Verification items for the finished model (mm, model axes). Coordinates: 2 decimals unless noted, no trailing zeros. Order: outer loops, then holes, each group sorted by start corner. A loop starts at its lowest first (then second) coordinate and runs counter-clockwise, first axis right, second up. Notation, with made-up numbers: (-17.5, 88.25) -> (5.5, 88.25) arc R15 ccw to (5.5, 115.25) -> close; hole circle Ø5 at (29, 25). An arc over 180 degrees is marked (long way). Use CSV: the item, a comma, the result in double quotes. Start each with the question number.
1) Scan lines: line 1 along X through (y, z) = (-20, 2.5); line 2 along Y through (x, z) = (0, 1.75); line 3 along X through (y, z) = (-8, 7.5). Record each from-to range of solid material in increasing order.
2) Go/stop test with flat-tipped pins: pin 1 (4 mm diameter, centred on x = 2.5, y = -19, fed in from +Z); pin 2 (5 mm diameter, centred on y = -15.5, z = 4.5, fed in from +X); pin 3 (6.5 mm diameter, centred on x = 1.5, y = 0, fed in from +Z); pin 4 (2 mm diameter, centred on x = 0, y = 0, fed in from +Z). Record where each tip stops, or that it passes through.
3) Sectioned sample at B-B on z = 3.5. Record the boundary of the cut face in (x, y).
from build123d import *
from OCP.BRepFilletAPI import BRepFilletAPI_MakeChamfer

# Parameters (mm, degrees)
SKETCH1_R                      = 30
SKETCH1_R_2                    = 28
SKETCH1_R_3                    = 4
BOSS_EXTRUDE1_DEPTH            = 2
BOSS_EXTRUDE2_START            = 8
SKETCH1_3_R                    = 4
BOSS_EXTRUDE2_DEPTH            = 8
BOSS_EXTRUDE3_START            = 28
SKETCH1_4_R                    = 30
BOSS_EXTRUDE3_DEPTH            = 28
CHAMFER1_SIZE2                 = 20
CHAMFER1_SIZE                  = 24
CIRPATTERN1_COUNT              = 4
CHAMFER1_OF_CIRPATTERN1_SIZE   = 24
CHAMFER1_OF_CIRPATTERN1_SIZE_2 = 20


with BuildPart() as part:
    # Sketch1 → Boss-Extrude1 (new body)
    # profile 1 of 6: a face of its own
    with BuildSketch(Plane.XY):
        Circle(SKETCH1_R)
        Circle(SKETCH1_R_2, mode=Mode.SUBTRACT)
    # profile 2 of 6: a face of its own
    with BuildSketch(Plane.XY):
        with BuildLine():
            Line((-0.75, 27.989953555), (-0.75, 3.929058411))
            ThreePointArc((-0.75, 3.929058411), (0, 4), (0.75, 3.929058411))
            Line((0.75, 3.929058411), (0.75, 27.989953555))
            ThreePointArc((0.75, 27.989953555), (0, 28), (-0.75, 27.989953555))
        make_face()
    # profile 3 of 6: a face of its own
    with BuildSketch(Plane.XY):
        with BuildLine():
            ThreePointArc((4, 0), (-2.549509757, -3.082207001), (-0.75, 3.929058411))
            Line((-0.75, 3.929058411), (-0.75, 27.989953555))
            ThreePointArc((-0.75, 27.989953555), (-19.532024985, -20.062402648), (28, 0))
            ThreePointArc((28, 0), (20.062402648, 19.532024985), (0.75, 27.989953555))
            Line((0.75, 27.989953555), (0.75, 3.929058411))
            ThreePointArc((0.75, 3.929058411), (3.082207001, 2.549509757), (4, 0))
        make_face()
    # profile 4 of 6: a face of its own
    with BuildSketch(Plane.XY):
        with BuildLine():
            ThreePointArc((4, 0), (-2.549509757, -3.082207001), (-0.75, 3.929058411))
            Line((-0.75, 3.929058411), (-0.75, 27.989953555))
            ThreePointArc((-0.75, 27.989953555), (-19.532024985, -20.062402648), (28, 0))
            ThreePointArc((28, 0), (20.062402648, 19.532024985), (0.75, 27.989953555))
            Line((0.75, 27.989953555), (0.75, 3.929058411))
            ThreePointArc((0.75, 3.929058411), (3.082207001, 2.549509757), (4, 0))
        make_face()
    # profile 5 of 6: a face of its own
    with BuildSketch(Plane.XY):
        with BuildLine():
            Line((-0.75, 27.989953555), (-0.75, 3.929058411))
            ThreePointArc((-0.75, 3.929058411), (0, 4), (0.75, 3.929058411))
            Line((0.75, 3.929058411), (0.75, 27.989953555))
            ThreePointArc((0.75, 27.989953555), (0, 28), (-0.75, 27.989953555))
        make_face()
    # profile 6 of 6: a face of its own
    with BuildSketch(Plane.XY):
        Circle(SKETCH1_R_3)
        with BuildLine():
            ThreePointArc((-1.25, 1.152171862), (0, -1.7), (1.25, 1.152171862))
            Line((1.25, 1.152171862), (-1.25, 1.152171862))
        make_face(mode=Mode.SUBTRACT)
    extrude(amount=-BOSS_EXTRUDE1_DEPTH)

    # Sketch1<3> → Boss-Extrude2 (add)
    with BuildSketch(Plane.XY.offset(BOSS_EXTRUDE2_START)):
        Circle(SKETCH1_3_R)
        with BuildLine():
            ThreePointArc((-1.25, 1.152171862), (0, -1.7), (1.25, 1.152171862))
            Line((1.25, 1.152171862), (-1.25, 1.152171862))
        make_face(mode=Mode.SUBTRACT)
    extrude(amount=-BOSS_EXTRUDE2_DEPTH)

    # Sketch1<4> → Boss-Extrude3 (add)
    with BuildSketch(Plane.XY.offset(BOSS_EXTRUDE3_START)):
        Circle(SKETCH1_4_R)
        with BuildLine():
            Line((-0.75, 27.989953555), (-0.75, 3.929058411))
            ThreePointArc((-0.75, 3.929058411), (0, 4), (0.75, 3.929058411))
            Line((0.75, 3.929058411), (0.75, 27.989953555))
            ThreePointArc((0.75, 27.989953555), (0, -28), (-0.75, 27.989953555))
        make_face(mode=Mode.SUBTRACT)
    boss_extrude3 = extrude(amount=-BOSS_EXTRUDE3_DEPTH)

    # Chamfer1
    chamfer1_edges = [part.edges().sort_by_distance(p)[0] for p in [
        (0, 4, 28),
    ]]
    chamfer1_side = [part.faces().sort_by_distance(p)[0] for p in [
        (0, 4.4, 28),
    ]]
    chamfer(chamfer1_edges, length=CHAMFER1_SIZE - 0.0001, length2=CHAMFER1_SIZE2 - 0.0001, reference=chamfer1_side[0])  # a hair under: the kernel refuses the full size

    # CirPattern1: Boss-Extrude3 ×4 about axis
    cirpattern1_axis = Axis((0, 0, 0), (0, 0, 1))
    for i in range(1, CIRPATTERN1_COUNT):
        add(boss_extrude3.rotate(cirpattern1_axis, i * 360 / CIRPATTERN1_COUNT))

    # Chamfer1 of CirPattern1
    chamfer1_of_cirpattern1_edges_1 = [part.edges().sort_by_distance(p)[0] for p in [
        (-4, 0, 28),
    ]]
    chamfer1_of_cirpattern1_side_1 = [part.faces().sort_by_distance(p)[0] for p in [
        (-4.4, 0, 28),
    ]]
    chamfer1_of_cirpattern1_edges_2 = [part.edges().sort_by_distance(p)[0] for p in [
        (0, -4, 28),
    ]]
    chamfer1_of_cirpattern1_side_2 = [part.faces().sort_by_distance(p)[0] for p in [
        (0, -4.4, 28),
    ]]
    chamfer1_of_cirpattern1_edges_3 = [part.edges().sort_by_distance(p)[0] for p in [
        (4, 0, 28),
    ]]
    chamfer1_of_cirpattern1_side_3 = [part.faces().sort_by_distance(p)[0] for p in [
        (4.4, 0, 28),
    ]]
    chamfer1_of_cirpattern1 = BRepFilletAPI_MakeChamfer(part.part.solid().wrapped)
    for e in chamfer1_of_cirpattern1_edges_1:
        chamfer1_of_cirpattern1.Add(CHAMFER1_OF_CIRPATTERN1_SIZE - 0.0001, CHAMFER1_OF_CIRPATTERN1_SIZE_2 - 0.0001, e.wrapped, chamfer1_of_cirpattern1_side_1[0].wrapped)
    for e in chamfer1_of_cirpattern1_edges_2:
        chamfer1_of_cirpattern1.Add(CHAMFER1_OF_CIRPATTERN1_SIZE - 0.0001, CHAMFER1_OF_CIRPATTERN1_SIZE_2 - 0.0001, e.wrapped, chamfer1_of_cirpattern1_side_2[0].wrapped)
    for e in chamfer1_of_cirpattern1_edges_3:
        chamfer1_of_cirpattern1.Add(CHAMFER1_OF_CIRPATTERN1_SIZE - 0.0001, CHAMFER1_OF_CIRPATTERN1_SIZE_2 - 0.0001, e.wrapped, chamfer1_of_cirpattern1_side_3[0].wrapped)
    add(Compound.cast(chamfer1_of_cirpattern1.Shape()), mode=Mode.REPLACE)  # a hair under: the kernel refuses the full size


solid = part.part
Answers follow:
1,line 1,"x = -22.36 to -19.6, -0.75 to 0.75, 19.6 to 22.36"
1,line 2,"y = -30 to -1.7, 1.15 to 30"
1,line 3,"x = -28.91 to -26.83, -0.75 to 0.75, 26.83 to 28.91"
2,pin 1,"stops at z = 21.32"
2,pin 2,"stops at x = 27.04"
2,pin 3,"stops at z = 8.63"
2,pin 4,"passes through"
3,outline,"circle Ø60 at (0, 0); hole (-27.99, -0.75) arc R28 ccw to (-0.75, -27.99) -> (-0.75, -3.93) arc R4 cw to (-3.93, -0.75) -> close; hole (-27.99, 0.75) -> (-3.93, 0.75) arc R4 cw to (-0.75, 3.93) -> (-0.75, 27.99) arc R28 ccw to start; hole (-1.25, 1.15) arc R1.7 ccw (long way) to (1.25, 1.15) -> close; hole (0.75, -27.99) arc R28 ccw to (27.99, -0.75) -> (3.93, -0.75) arc R4 cw to (0.75, -3.93) -> close; hole (0.75, 3.93) arc R4 cw to (3.93, 0.75) -> (27.99, 0.75) arc R28 ccw to (0.75, 27.99) -> close"
